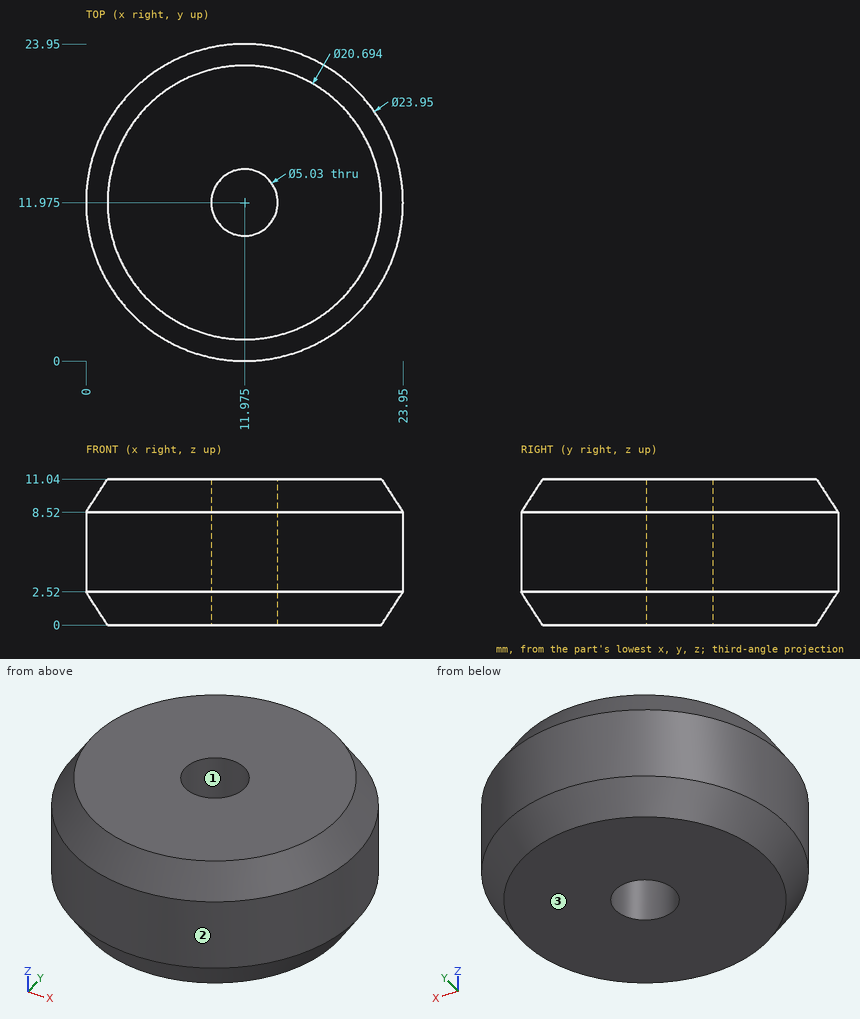
For this review, use the dimensioned drawing (mm, ordinates from the lowest corner) and the shaded views. Give positions to 0.01 mm unless a question says otherwise; leave off trailing zeros.
(1) The part is to be moulded in two halves that separate along Y. For the marked faces 1, 2 and 3, say which applies: released by +Y, released by -Y, zero draft, split by the parting line, or undercut.
(2) For P1, Ø3, axis at x = 9, z = 1.5, coming from the -Y side; P2, Ø1, axis at x = 12.5, z = 9.5, coming from the -Y side; P3, Ø6, axis at y = 6, z = 1.5, coming from the -X side; P4, Ø3, axis at x = 11.975, y = 11.975, coming from the +Z side, all flat-tipped, find the tip position at first contact; note any pin that passes through.
(3) To check wall thickness, follow L1, parallel to X at y = 19.75, z = 8 (1 decimal); L2, parallel to Y at x = 1, z = 6.25 (1 decimal); L3, parallel to X at y = 18, z = 5.5 (1 decimal). State the ranges of each line that lie inside material, in increasing order.
Returned:
1. face 1: undercut
1. face 2: split by the parting line
1. face 3: zero draft
2. P1: stops at y = 0.15
2. P2: stops at y = 0.32
2. P3: stops at x = 0.42
2. P4: passes through
3. L1: x = 2.9 to 21.1
3. L2: y = 7.2 to 16.8
3. L3: x = 1.6 to 22.3
